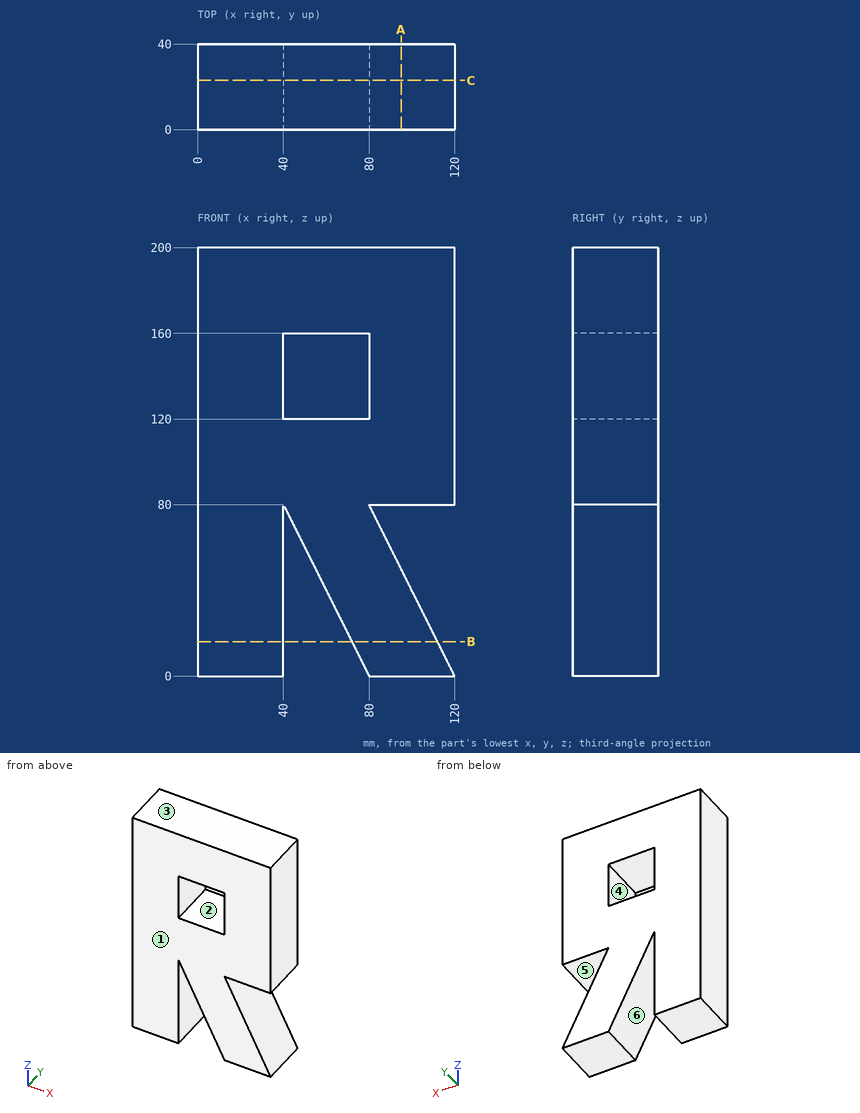
Geometry: see drawing. Coordinates: mm, zero at the bounding-box minimum. A direction names the side the tool comes from. Round coordinates to 2 decimals unless told otherwise and drop trailing zeros. Loops run counter-clockwise (first coordinate to the right, second up) from the corner with the lowest first, then second, coordinate; pieces in that order, holes last.
(1) Access query for the marked faces 4, 5 and 6. Directions: +Z, -Z, +X, -X, +Y, -Y. A direction counts if a zero-diameter tool reaches every point of the face in a straight line with its end or side. Return the directions, or none.
From the geometry:
face 4: +Y, -Y
face 5: +X, +Y, -Y
face 6: -Z, +Y, -Y
(2) Section query C-C (y = 23). Output: boundary loops of the cut face in (x, z), and give its area (3 significant figures).
From the geometry:
outline: (0, 0) - (40, 0) - (40, 80) - (80, 0) - (120, 0) - (80, 80) - (120, 80) - (120, 200) - (0, 200) - close; hole (40, 120) - (80, 120) - (80, 160) - (40, 160) - close
area: 19,200 mm2
(3) Contact query for flat-ended pins moving along their axis: pin 1 Ø12 at (x, y) = (63.5, 22.5) entering from -Z; pin 2 Ø12 at (y, z) = (19.5, 53) entering from +X; pin 3 Ø6 at (y, z) = (10.5, 71.5) entering from +X. Output: stop coordinate, or through.
From the geometry:
pin 1: stops at z = 21
pin 2: stops at x = 96.5
pin 3: stops at x = 85.75
(4) Section query B-B (z = 16). Output: boundary loops of the cut face in (x, y).
From the geometry:
outline: (0, 0) - (40, 0) - (40, 40) - (0, 40) - close; (72, 0) - (112, 0) - (112, 40) - (72, 40) - close
(5) Material intervals for probe 1 along X at (y, z) = (12, 159.5); probe 2 along Z at (x, y) = (60, 28); probe 3 along Z at (x, y) = (100, 23.5), sorted ascending.
From the geometry:
probe 1: x = 0 to 40, 80 to 120
probe 2: z = 40 to 120, 160 to 200
probe 3: z = 0 to 40, 80 to 200
(6) Section query A-A (x = 95). Output: boundary loops of the cut face in (y, z).
From the geometry:
outline: (0, 0) - (40, 0) - (40, 50) - (0, 50) - close; (0, 80) - (40, 80) - (40, 200) - (0, 200) - close
(7) Pull-direction query (Z, two-part tool) for the marked faces 1, 2 and 3; classes: +Z half, -Z half, draft (parallel to the pull), parting line (faces both ways), or undercut.
From the geometry:
face 1: draft
face 2: undercut
face 3: +Z half
